from build123d import *

# Parameters (mm, degrees)
SKETCH1_W               = 50.8
SKETCH1_H               = 31.75
BOSS_EXTRUDE1_DEPTH     = 31.75
SKETCH2_W               = 25.4
SKETCH2_H               = 25.4
CUT_EXTRUDE1_DEPTH      = 85.79053849
SKETCH3_W               = 6.35
SKETCH3_H               = 31.75
BOSS_EXTRUDE2_DEPTH     = 19.05
SKETCH4_W               = 6.35
SKETCH4_H               = 31.75
BOSS_EXTRUDE3_DEPTH     = 19.05
CUT_EXTRUDE2_DEPTH      = 91.317082645
CUT_EXTRUDE2_DEPTH_BACK = 91.317082645
SKETCH5_R               = 3.175
FILLET1_R               = 3
SKETCH6_R               = 3.429
CUT_EXTRUDE3_DEPTH      = 126.026704643
SKETCH7_R               = 3.429
CUT_EXTRUDE4_DEPTH      = 126.026704643


with BuildPart() as part:
    # Sketch1 → Boss-Extrude1 (new body)
    with BuildSketch(Plane(origin=(0, 0, 0), x_dir=(1, 0, 0), z_dir=(0, 1, 0))):
        with Locations((-84.340486484, 44.131107335)):
            Rectangle(SKETCH1_W, SKETCH1_H)
    extrude(amount=BOSS_EXTRUDE1_DEPTH)

    # Sketch2 → Cut-Extrude1 (cut, through all)
    with BuildSketch(Plane(origin=(-58.940486484, 0, 0), x_dir=(0, 0, -1), z_dir=(1, 0, 0))):
        with Locations((44.131107335, 12.7)):
            Rectangle(SKETCH2_W, SKETCH2_H)
    extrude(amount=-CUT_EXTRUDE1_DEPTH, mode=Mode.SUBTRACT)

    # Sketch3 → Boss-Extrude2 (add)
    with BuildSketch(Plane(origin=(0, 31.75, 0), x_dir=(1, 0, 0), z_dir=(0, 1, 0))):
        with Locations((-106.565486484, 44.131107335)):
            Rectangle(SKETCH3_W, SKETCH3_H)
    extrude(amount=BOSS_EXTRUDE2_DEPTH)

    # Sketch4 → Boss-Extrude3 (add)
    with BuildSketch(Plane(origin=(0, 31.75, 0), x_dir=(1, 0, 0), z_dir=(0, 1, 0))):
        with Locations((-62.115486484, 44.131107335)):
            Rectangle(SKETCH4_W, SKETCH4_H)
    extrude(amount=BOSS_EXTRUDE3_DEPTH)

    # Sketch5 → Cut-Extrude2 (cut, two sides: drawn at the far end of the back side and taken through both)
    with BuildSketch(Plane(origin=(-103.390486484, 0, 0), x_dir=(0, 0, -1), z_dir=(1, 0, 0)).offset(-CUT_EXTRUDE2_DEPTH_BACK)):
        with Locations((44.053057169, 41.275)):
            Circle(SKETCH5_R)
    extrude(amount=CUT_EXTRUDE2_DEPTH + CUT_EXTRUDE2_DEPTH_BACK, mode=Mode.SUBTRACT)

    # Fillet1
    fillet1_edges = [part.edges().sort_by_distance(p)[0] for p in [
        (-106.565486484, 50.8, -60.006107335),
        (-106.565486484, 50.8, -28.256107335),
        (-62.115486484, 50.8, -28.256107335),
        (-62.115486484, 50.8, -60.006107335),
        (-65.290486484, 31.75, -44.131107335),
        (-103.390486484, 31.75, -44.131107335),
    ]]
    fillet(fillet1_edges, radius=FILLET1_R)

    # Sketch6 → Cut-Extrude3 (cut, through all)
    with BuildSketch(Plane(origin=(0, 0, -60.006107335), x_dir=(-1, 0, 0), z_dir=(0, 0, -1))):
        with Locations((68.290486484, 12.7)):
            Circle(SKETCH6_R)
    extrude(amount=-CUT_EXTRUDE3_DEPTH, mode=Mode.SUBTRACT)

    # Sketch7 → Cut-Extrude4 (cut, through all)
    with BuildSketch(Plane(origin=(0, 0, -60.006107335), x_dir=(-1, 0, 0), z_dir=(0, 0, -1))):
        with Locations((100.390486484, 12.7)):
            Circle(SKETCH7_R)
    extrude(amount=-CUT_EXTRUDE4_DEPTH, mode=Mode.SUBTRACT)


solid = part.part
The model under review builds one solid part; all positions refer to its coordinate system, in mm. A direction names the side the tool comes from. Give positions to 0.01 mm unless a question says otherwise; leave off trailing zeros. Loops run counter-clockwise (first coordinate to the right, second up) from the corner with the lowest first, then second, coordinate; pieces in that order, holes last. Notation, with made-up numbers: (60, 75) -> (78, 75) arc R10 ccw to (78, 93) -> close; hole circle Ø6 at (69.5, -12). An arc over 180 degrees is marked (long way). Put each result on its own line as item: value. Start each with the question number.
1. Clearance check with flat-ended pins moving along their axes: P1, Ø5.5, axis at y = 41.28, z = -44.05, coming from the -X side; P2, Ø2, axis at x = -87.5, z = -48, coming from the +Y side; P3, Ø12.5, axis at x = -87, z = -40.5, coming from the -Y side. State where each tip first meets the part, or that it passes through.
2. We need section C-C on x = -63.5. State the section outline as (y, z) points (3 decimals).
3. We need section B-B on z = -42. State the section outline as (x, y) points.
4. Mouldability with a two-part tool opening along Y and no side actions: class faces 1 (the face through (-102.488, 32.605, -44.353)), 2 (the face through (-64.865, 12.851, -58.441)), 3 (the face through (-103.39, 46, -44)) as released by +Y, released by -Y, zero draft, split by the parting line, or undercut.
5. We need section D-D on y = 12.7. State the section outline as (x, z) points.
6. For faces 4 (the face through (-84, 25.4, -44)), 5 (the face through (-103.56, 11.39, -29.87)), 6 (the face through (-65.29, 46, -44)), list the 3-axis set-ups (+Z, -Z, +X, -X, +Y, -Y) from which the entire face can be reached by the end or side of a thin tool; tool diameter is ignored.
7. Wall thickness on probe 1 along Z at (x, y) = (-107, 10); probe 2 along X at (y, z) = (47.5, -37.5); probe 3 along Y at (x, z) = (-70.5, -55): over which ranges is each line inside the solid? List them lowest first.
8. We need section A-A on y = 23. State the section outline as (x, z) points, then the cut area to 3 significant figures.
Determined:
1. P1: through
1. P2: y = 31.75
1. P3: y = 25.4
2. outline: (0, -60.006) -> (47.8, -60.006) arc R3 ccw to (50.8, -57.006) -> (50.8, -31.256) arc R3 ccw to (47.8, -28.256) -> (0, -28.256) -> (0, -31.431) -> (25.4, -31.431) -> (25.4, -56.831) -> (0, -56.831) -> close; hole circle Ø6.35 at (41.275, -44.053)
3. outline: (-109.74, 25.4) -> (-58.94, 25.4) -> (-58.94, 38.85) -> (-65.29, 38.85) -> (-65.29, 34.75) arc R3 cw to (-68.29, 31.75) -> (-100.39, 31.75) arc R3 cw to (-103.39, 34.75) -> (-103.39, 38.85) -> (-109.74, 38.85) -> close; (-109.74, 43.7) -> (-103.39, 43.7) -> (-103.39, 50.8) -> (-109.74, 50.8) -> close; (-65.29, 43.7) -> (-58.94, 43.7) -> (-58.94, 50.8) -> (-65.29, 50.8) -> close
4. face 1: released by +Y
4. face 2: undercut
4. face 3: zero draft
5. outline: (-109.74, -60.01) -> (-103.82, -60.01) -> (-103.82, -56.83) -> (-109.74, -56.83) -> close; (-109.74, -31.43) -> (-103.82, -31.43) -> (-103.82, -28.26) -> (-109.74, -28.26) -> close; (-96.96, -60.01) -> (-71.72, -60.01) -> (-71.72, -56.83) -> (-96.96, -56.83) -> close; (-96.96, -31.43) -> (-71.72, -31.43) -> (-71.72, -28.26) -> (-96.96, -28.26) -> close; (-64.86, -60.01) -> (-58.94, -60.01) -> (-58.94, -56.83) -> (-64.86, -56.83) -> close; (-64.86, -31.43) -> (-58.94, -31.43) -> (-58.94, -28.26) -> (-64.86, -28.26) -> close
6. face 4: +X, -X, -Y
6. face 5: +Z, -Z
6. face 6: +Z, -Z, +Y
7. probe 1: -60.01 to -56.83, -31.43 to -28.26
7. probe 2: -109.74 to -103.39, -65.29 to -58.94
7. probe 3: 25.4 to 31.75
8. outline: (-109.74, -60.01) -> (-58.94, -60.01) -> (-58.94, -56.83) -> (-109.74, -56.83) -> close; (-109.74, -31.43) -> (-58.94, -31.43) -> (-58.94, -28.26) -> (-109.74, -28.26) -> close
8. area: 323 mm^2
